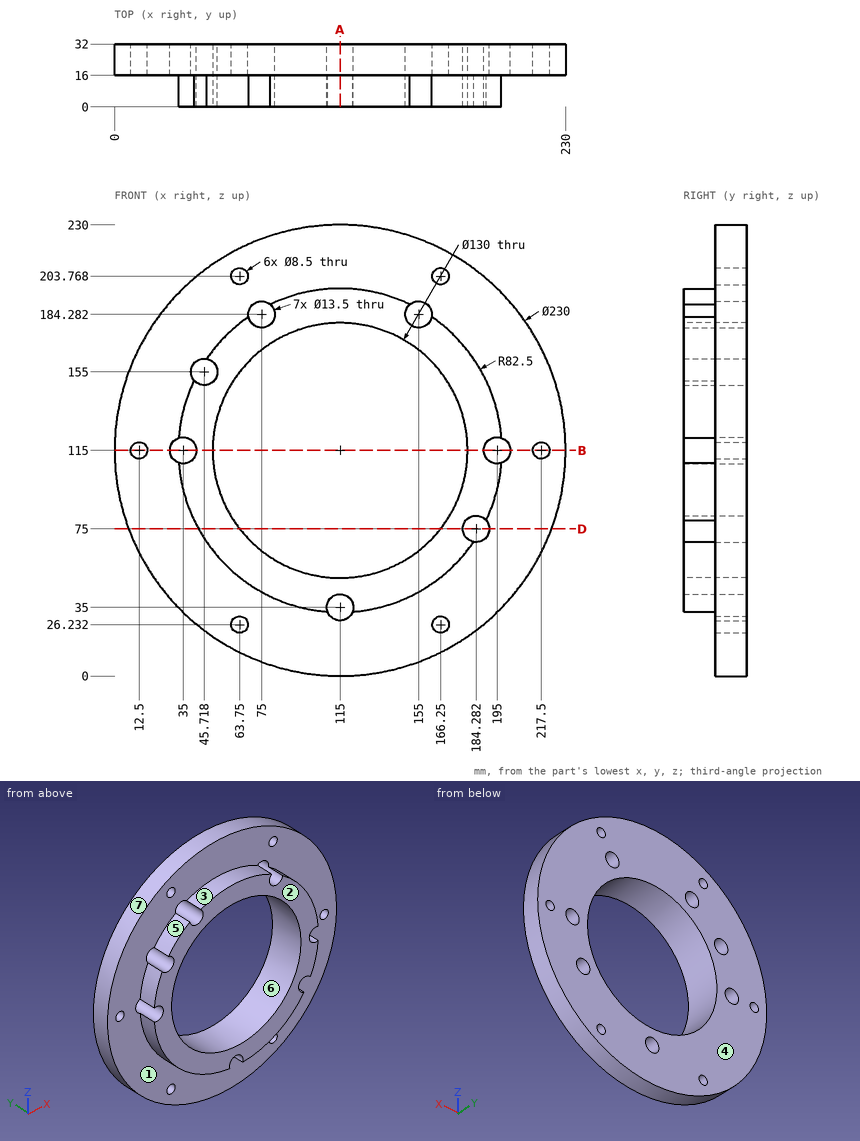
For this review, use the dimensioned drawing (mm, ordinates from the lowest corner) and the shaded views. A direction names the side the tool comes from. Coordinates: 2 decimals unless noted, no trailing zeros. Loops run counter-clockwise (first coordinate to the right, second up) from the corner with the lowest first, then second, coordinate; pieces in that order, holes last. Notation, with made-up numbers: (2, 30.5) -> (42, 30.5) arc R18 cw to (42, 56.5) -> close; hole circle Ø3 at (-19.75, -31.75). An arc over 180 degrees is marked (long way). Use a Markdown table: item, result. Add a question column.
Item 1: We need section A-A, the plane x = 115. Write out the cut boundary in (y, z), and give its area (3 significant figures).
Item 2: Machinability: for the marked faces 1, 2 and 3, which of the approach directions +Z, -Z, +X, -X, +Y, -Y give a long, thin tool a straight path to every point of the face, cutting with its end or side? Answer none if there is none.
Item 3: The part is to be moulded in two halves that separate along X. For the marked faces 4, 5, 6 and 7, say which applies: +X half, -X half, draft (parallel to the pull), parting line (faces both ways), or undercut.
Item 4: Clearance check with flat-ended pins moving along their axes: P1, Ø7, axis at x = 166.25, z = 26.23, coming from the -Y side; P2, Ø5, axis at x = 36, y = 28, coming from the +Z side (1 decimal); P3, Ø1, axis at x = 28, y = 25.5, coming from the -Z side; P4, Ø10, axis at y = 22, z = 59, coming from the +X side. State where each tip first meets the part, or that it passes through.
Item 5: Wall thickness on L1, parallel to X at y = 17, z = 75 (1 decimal); L2, parallel to X at y = 17, z = 184.5 (1 decimal); L3, parallel to X at y = 19, z = 113: over which ranges is each line inside the solid? List them lowest first. Write a range as from..to.
Item 6: We need section B-B, the plane z = 115. Write out the cut boundary in (x, y).
Item 7: We need section D-D, the plane z = 75. Write out the cut boundary in (x, y) (1 decimal), and give its area (3 significant figures).
Numbers:
| question | item | result |
|---|---|---|
| 1 | outline | (0, 41.75) -> (32, 41.75) -> (32, 50) -> (0, 50) -> close; (0, 180) -> (32, 180) -> (32, 230) -> (16, 230) -> (16, 197.5) -> (0, 197.5) -> close; (16, 0) -> (32, 0) -> (32, 28.25) -> (16, 28.25) -> close |
| 1 | area | 1,800 mm^2 |
| 2 | face 1 | -Y |
| 2 | face 2 | +Z, -Z, +X, -X, -Y |
| 2 | face 3 | +Z, -Y |
| 3 | face 4 | draft |
| 3 | face 5 | -X half |
| 3 | face 6 | undercut |
| 3 | face 7 | parting line |
| 4 | P1 | passes through |
| 4 | P2 | stops at z = 200.9 |
| 4 | P3 | stops at z = 39.22 |
| 4 | P4 | stops at x = 218.07 |
| 5 | L1 | x = 7.2..63.8, 166.2..177.5, 191..222.8 |
| 5 | L2 | x = 23.4..68.3, 81.7..148.3, 161.7..206.6 |
| 5 | L3 | x = 0.02..8.75, 16.25..28.55, 41.45..50.03, 179.97..188.55, 201.45..213.75, 221.25..229.98 |
| 6 | outline | (0, 16) -> (8.25, 16) -> (8.25, 32) -> (0, 32) -> close; (16.75, 16) -> (28.25, 16) -> (28.25, 32) -> (16.75, 32) -> close; (41.75, 0) -> (50, 0) -> (50, 32) -> (41.75, 32) -> close; (180, 0) -> (188.25, 0) -> (188.25, 32) -> (180, 32) -> close; (201.75, 16) -> (213.25, 16) -> (213.25, 32) -> (201.75, 32) -> close; (221.75, 16) -> (230, 16) -> (230, 32) -> (221.75, 32) -> close |
| 7 | outline | (7.2, 16) -> (42.8, 16) -> (42.8, 0) -> (63.8, 0) -> (63.8, 32) -> (7.2, 32) -> close; (166.2, 0) -> (177.5, 0) -> (177.5, 32) -> (166.2, 32) -> close; (191, 16) -> (222.8, 16) -> (222.8, 32) -> (191, 32) -> close |
| 7 | area | 2,110 mm^2 |
